Work out the finished part from the listing and answer in its coordinate system (mm). Face numbers are marked on the shaded views. A direction names the side the tool comes from. Round coordinates to 2 decimals unless told otherwise and drop trailing zeros. Loops run counter-clockwise (first coordinate to the right, second up) from the corner with the lowest first, then second, coordinate; pieces in that order, holes last. Notation, with made-up numbers: (19.5, 70.25) -> (31.5, 70.25) arc R13 cw to (31.5, 91.25) -> close; hole circle Ø3 at (38, 84). An arc over 180 degrees is marked (long way). Use one line per item in the form item = value.
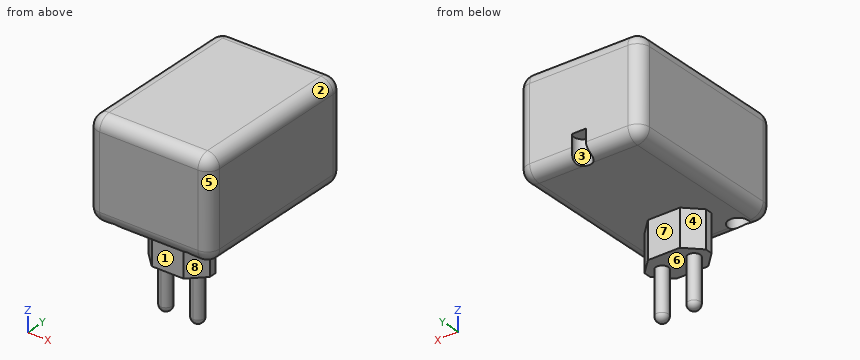
```python
from build123d import *

# Parameters (mm, degrees)
F0_W          = 50
F0_H          = 70
F1_DEPTH      = 40
F3_DEPTH      = 15
F4_SIZE       = 6
F6_DEPTH      = 20
F7_DEPTH      = 20
F8_R          = 2.5
F10_DEPTH     = 10
F12_DEPTH     = 8
F13_T1_DEPTH  = 60
F13_T3_DEPTH  = 30
F13_T5_DEPTH  = 29.6276373277
F13_T7_DEPTH  = 29.6276373277
F13_T9_DEPTH  = 40
F13_S13_W     = 5
F13_S13_H     = 5
F13_T14_DEPTH = 5
F13_S19_W     = 5
F13_S19_H     = 5
F13_T20_DEPTH = 5
F13_S25_W     = 5
F13_S25_H     = 5
F13_T26_DEPTH = 5
F13_S31_W     = 5
F13_S31_H     = 5
F13_T32_DEPTH = 5
F13_S37_W     = 5
F13_S37_H     = 5
F13_T38_DEPTH = 5
F13_S43_W     = 5
F13_S43_H     = 5
F13_T44_DEPTH = 5
F13_S49_W     = 5
F13_S49_H     = 5
F13_T50_DEPTH = 5
F13_S55_W     = 5
F13_S55_H     = 5
F13_T56_DEPTH = 5


# Not quite as in the source:
# - a fillet or chamfer that OpenCascade refuses, or shapes differently, is made with other operations: its cross-section is extruded or revolved along the edge and cut away or added


with BuildPart() as f1:
    # F0 (on Top) → F1 (new body)
    with BuildSketch(Plane.XY):
        Rectangle(F0_W, F0_H)
    extrude(amount=F1_DEPTH)

    # F2 (on face) → F3 (join)
    with BuildSketch(Plane(origin=(0, 0, 0), x_dir=(1, 0, 0), z_dir=(0, 0, -1))):
        Polygon((-12.5, 25), (-12.5, 20), (-12.5, 10), (12.5, 10), (12.5, 17.5), (12.5, 25), align=None)
    extrude(amount=F3_DEPTH)

    # F4
    f4_edges = [f1.edges().sort_by_distance(p)[0] for p in [
        (-12.5, -25, -7.5),
        (-12.5, -10, -7.5),
        (12.5, -10, -7.5),
        (12.5, -25, -7.5),
    ]]
    chamfer(f4_edges, length=F4_SIZE)

    # F5 (on face) → F6 (join)
    with BuildSketch(Plane(origin=(0, 0, -15), x_dir=(1, 0, 0), z_dir=(0, 0, -1))):
        with BuildLine():
            ThreePointArc((-4, 17.5), (-4.732233047, 19.267766953), (-6.5, 20))
            ThreePointArc((-6.5, 20), (-8.267766953, 15.732233047), (-4, 17.5))
        make_face()
    extrude(amount=F6_DEPTH)

    # F5 (on face) → F7 (join)
    with BuildSketch(Plane(origin=(0, 0, -15), x_dir=(1, 0, 0), z_dir=(0, 0, -1))):
        with BuildLine():
            ThreePointArc((9, 17.5), (8.267766953, 19.267766953), (6.5, 20))
            ThreePointArc((6.5, 20), (4.732233047, 15.732233047), (9, 17.5))
        make_face()
    extrude(amount=F7_DEPTH)

    # F8
    f8_edges = [f1.edges().sort_by_distance(p)[0] for p in [
        (-9, -17.5, -35),
        (4, -17.5, -35),
    ]]
    fillet(f8_edges, radius=F8_R)

    # F9 (on face) → F10 (cut)
    with BuildSketch(Plane(origin=(0, 0, 0), x_dir=(1, 0, 0), z_dir=(0, 0, -1))):
        with BuildLine():
            Line((-2.8723626723, -35), (2.8723626723, -35))
            ThreePointArc((2.8723626723, -35), (0, -29.4152137969), (-2.8723626723, -35))
        make_face()
    extrude(amount=-F10_DEPTH, mode=Mode.SUBTRACT)

    # F11 (on face) → F12 (cut)
    with BuildSketch(Plane(origin=(0, 0, 0), x_dir=(1, 0, 0), z_dir=(0, 0, -1))):
        with BuildLine():
            ThreePointArc((11, 29.8445560038), (15, 25.8445560038), (19, 29.8445560038))
            Line((19, 29.8445560038), (15, 29.8445560038))
            Line((15, 29.8445560038), (11, 29.8445560038))
        make_face()
        with BuildLine():
            Line((-15, 29.8445560038), (-11, 29.8445560038))
            ThreePointArc((-11, 29.8445560038), (-15, 33.8445560038), (-19, 29.8445560038))
            Line((-19, 29.8445560038), (-15, 29.8445560038))
        make_face()
        with BuildLine():
            ThreePointArc((-19, 29.8445560038), (-15, 25.8445560038), (-11, 29.8445560038))
            Line((-11, 29.8445560038), (-15, 29.8445560038))
            Line((-15, 29.8445560038), (-19, 29.8445560038))
        make_face()
        with BuildLine():
            Line((15, 29.8445560038), (19, 29.8445560038))
            ThreePointArc((19, 29.8445560038), (15, 33.8445560038), (11, 29.8445560038))
            Line((11, 29.8445560038), (15, 29.8445560038))
        make_face()
    extrude(amount=-F12_DEPTH, mode=Mode.SUBTRACT)

    # F13: fillet of radius 5 on 13 edges, made by hand

    # F13_s2 → F13_t1 (cut)
    with BuildSketch(Plane.XZ.offset(-30)):
        with BuildLine():
            ThreePointArc((20, 0), (23.5355339059, 1.4644660941), (25, 5))
            Line((25, 5), (25, 0))
            Line((25, 0), (20, 0))
        make_face()
        with BuildLine():
            ThreePointArc((25, 35), (23.5355339059, 38.5355339059), (20, 40))
            Line((20, 40), (25, 40))
            Line((25, 40), (25, 35))
        make_face()
        with BuildLine():
            ThreePointArc((-20, 0), (-23.5355339059, 1.4644660941), (-25, 5))
            Line((-25, 5), (-25, 0))
            Line((-25, 0), (-20, 0))
        make_face()
        with BuildLine():
            ThreePointArc((-25, 35), (-23.5355339059, 38.5355339059), (-20, 40))
            Line((-20, 40), (-25, 40))
            Line((-25, 40), (-25, 35))
        make_face()
    extrude(amount=F13_T1_DEPTH, mode=Mode.SUBTRACT)

    # F13_s4 → F13_t3 (cut)
    with BuildSketch(Plane.XY.offset(5)):
        with BuildLine():
            ThreePointArc((20, -35), (23.5355339059, -33.5355339059), (25, -30))
            Line((25, -30), (25, -35))
            Line((25, -35), (20, -35))
        make_face()
        with BuildLine():
            ThreePointArc((20, 35), (23.5355339059, 33.5355339059), (25, 30))
            Line((25, 30), (25, 35))
            Line((25, 35), (20, 35))
        make_face()
        with BuildLine():
            ThreePointArc((-25, -30), (-23.5355339059, -33.5355339059), (-20, -35))
            Line((-20, -35), (-25, -35))
            Line((-25, -35), (-25, -30))
        make_face()
        with BuildLine():
            ThreePointArc((-25, 30), (-23.5355339059, 33.5355339059), (-20, 35))
            Line((-20, 35), (-25, 35))
            Line((-25, 35), (-25, 30))
        make_face()
    extrude(amount=F13_T3_DEPTH, mode=Mode.SUBTRACT)

    # F13_s6 → F13_t5 (cut)
    with BuildSketch(Plane.YZ.offset(-9.6276373277)):
        with BuildLine():
            ThreePointArc((30, 0), (33.5355339059, 1.4644660941), (35, 5))
            Line((35, 5), (35, 0))
            Line((35, 0), (30, 0))
        make_face()
    extrude(amount=F13_T5_DEPTH, mode=Mode.SUBTRACT)

    # F13_s8 → F13_t7 (cut)
    with BuildSketch(Plane.YZ.offset(-20)):
        with BuildLine():
            ThreePointArc((30, 0), (33.5355339059, 1.4644660941), (35, 5))
            Line((35, 5), (35, 0))
            Line((35, 0), (30, 0))
        make_face()
    extrude(amount=F13_T7_DEPTH, mode=Mode.SUBTRACT)

    # F13_s10 → F13_t9 (cut)
    with BuildSketch(Plane.YZ.offset(-20)):
        with BuildLine():
            ThreePointArc((-30, 0), (-33.5355339059, 1.4644660941), (-35, 5))
            Line((-35, 5), (-35, 0))
            Line((-35, 0), (-30, 0))
        make_face()
        with BuildLine():
            ThreePointArc((-35, 35), (-33.5355339059, 38.5355339059), (-30, 40))
            Line((-30, 40), (-35, 40))
            Line((-35, 40), (-35, 35))
        make_face()
        with BuildLine():
            ThreePointArc((35, 35), (33.5355339059, 38.5355339059), (30, 40))
            Line((30, 40), (35, 40))
            Line((35, 40), (35, 35))
        make_face()
    extrude(amount=F13_T9_DEPTH, mode=Mode.SUBTRACT)


with BuildPart() as f13_tool12:
    # F13_s13 → F13_t14 (new body)
    with BuildSketch(Plane.XZ.offset(30)):
        with Locations((22.5, 2.5)):
            Rectangle(F13_S13_W, F13_S13_H)
    extrude(amount=F13_T14_DEPTH)

    # F13_s15 → F13_t16 (revolve, cut)
    with BuildSketch(Plane(origin=(20, -30, 5), x_dir=(-0.7071067812, 0, 0.7071067812), z_dir=(0.7071067812, 0, 0.7071067812))):
        with BuildLine():
            ThreePointArc((0, -5), (5, 0), (0, 5))
            Line((0, 5), (0, -5))
        make_face()
    revolve(axis=Axis((20, -30, 5), (0, -1, 0)), mode=Mode.SUBTRACT)


with BuildPart() as f1_1:
    add(f1.part)

    # F13_t11: cut F13_tool12
    add(f13_tool12.part, mode=Mode.SUBTRACT)


with BuildPart() as f13_tool18:
    # F13_s19 → F13_t20 (new body)
    with BuildSketch(Plane.YZ.offset(20)):
        with Locations((32.5, 2.5)):
            Rectangle(F13_S19_W, F13_S19_H)
    extrude(amount=F13_T20_DEPTH)

    # F13_s21 → F13_t22 (revolve, cut)
    with BuildSketch(Plane(origin=(20, 30, 5), x_dir=(0, -0.7071067812, 0.7071067812), z_dir=(0, 0.7071067812, 0.7071067812))):
        with BuildLine():
            ThreePointArc((0, -5), (5, 0), (0, 5))
            Line((0, 5), (0, -5))
        make_face()
    revolve(axis=Axis((20, 30, 5), (1, 0, 0)), mode=Mode.SUBTRACT)


with BuildPart() as f1_2:
    add(f1_1.part)

    # F13_t17: cut F13_tool18
    add(f13_tool18.part, mode=Mode.SUBTRACT)


with BuildPart() as f13_tool24:
    # F13_s25 → F13_t26 (new body)
    with BuildSketch(Plane.XZ.offset(30)):
        with Locations((22.5, 37.5)):
            Rectangle(F13_S25_W, F13_S25_H)
    extrude(amount=F13_T26_DEPTH)

    # F13_s27 → F13_t28 (revolve, cut)
    with BuildSketch(Plane(origin=(20, -30, 35), x_dir=(-0.7071067812, 0, -0.7071067812), z_dir=(-0.7071067812, 0, 0.7071067812))):
        with BuildLine():
            ThreePointArc((0, -5), (5, 0), (0, 5))
            Line((0, 5), (0, -5))
        make_face()
    revolve(axis=Axis((20, -30, 35), (0, -1, 0)), mode=Mode.SUBTRACT)


with BuildPart() as f1_3:
    add(f1_2.part)

    # F13_t23: cut F13_tool24
    add(f13_tool24.part, mode=Mode.SUBTRACT)


with BuildPart() as f13_tool30:
    # F13_s31 → F13_t32 (new body)
    with BuildSketch(Plane.YZ.offset(20)):
        with Locations((32.5, 37.5)):
            Rectangle(F13_S31_W, F13_S31_H)
    extrude(amount=F13_T32_DEPTH)

    # F13_s33 → F13_t34 (revolve, cut)
    with BuildSketch(Plane(origin=(20, 30, 35), x_dir=(0, -0.7071067812, -0.7071067812), z_dir=(0, -0.7071067812, 0.7071067812))):
        with BuildLine():
            ThreePointArc((0, -5), (5, 0), (0, 5))
            Line((0, 5), (0, -5))
        make_face()
    revolve(axis=Axis((20, 30, 35), (1, 0, 0)), mode=Mode.SUBTRACT)


with BuildPart() as f1_4:
    add(f1_3.part)

    # F13_t29: cut F13_tool30
    add(f13_tool30.part, mode=Mode.SUBTRACT)


with BuildPart() as f13_tool36:
    # F13_s37 → F13_t38 (new body)
    with BuildSketch(Plane.XY.offset(5)):
        with Locations((-22.5, 32.5)):
            Rectangle(F13_S37_W, F13_S37_H)
    extrude(amount=-F13_T38_DEPTH)

    # F13_s39 → F13_t40 (revolve, cut)
    with BuildSketch(Plane(origin=(-20, 30, 5), x_dir=(0.7071067812, -0.7071067812, 0), z_dir=(0.7071067812, 0.7071067812, 0))):
        with BuildLine():
            ThreePointArc((0, -5), (5, 0), (0, 5))
            Line((0, 5), (0, -5))
        make_face()
    revolve(axis=Axis((-20, 30, 5), (0, 0, -1)), mode=Mode.SUBTRACT)


with BuildPart() as f1_5:
    add(f1_4.part)

    # F13_t35: cut F13_tool36
    add(f13_tool36.part, mode=Mode.SUBTRACT)


with BuildPart() as f13_tool42:
    # F13_s43 → F13_t44 (new body)
    with BuildSketch(Plane.XZ.offset(30)):
        with Locations((-22.5, 2.5)):
            Rectangle(F13_S43_W, F13_S43_H)
    extrude(amount=F13_T44_DEPTH)

    # F13_s45 → F13_t46 (revolve, cut)
    with BuildSketch(Plane(origin=(-20, -30, 5), x_dir=(0.7071067812, 0, 0.7071067812), z_dir=(0.7071067812, 0, -0.7071067812))):
        with BuildLine():
            ThreePointArc((0, -5), (5, 0), (0, 5))
            Line((0, 5), (0, -5))
        make_face()
    revolve(axis=Axis((-20, -30, 5), (0, -1, 0)), mode=Mode.SUBTRACT)


with BuildPart() as f1_6:
    add(f1_5.part)

    # F13_t41: cut F13_tool42
    add(f13_tool42.part, mode=Mode.SUBTRACT)


with BuildPart() as f13_tool48:
    # F13_s49 → F13_t50 (new body)
    with BuildSketch(Plane.XZ.offset(30)):
        with Locations((-22.5, 37.5)):
            Rectangle(F13_S49_W, F13_S49_H)
    extrude(amount=F13_T50_DEPTH)

    # F13_s51 → F13_t52 (revolve, cut)
    with BuildSketch(Plane(origin=(-20, -30, 35), x_dir=(0.7071067812, 0, -0.7071067812), z_dir=(-0.7071067812, 0, -0.7071067812))):
        with BuildLine():
            ThreePointArc((0, -5), (5, 0), (0, 5))
            Line((0, 5), (0, -5))
        make_face()
    revolve(axis=Axis((-20, -30, 35), (0, -1, 0)), mode=Mode.SUBTRACT)


with BuildPart() as f1_7:
    add(f1_6.part)

    # F13_t47: cut F13_tool48
    add(f13_tool48.part, mode=Mode.SUBTRACT)


with BuildPart() as f13_tool54:
    # F13_s55 → F13_t56 (new body)
    with BuildSketch(Plane.XY.offset(35)):
        with Locations((-22.5, 32.5)):
            Rectangle(F13_S55_W, F13_S55_H)
    extrude(amount=F13_T56_DEPTH)

    # F13_s57 → F13_t58 (revolve, cut)
    with BuildSketch(Plane(origin=(-20, 30, 35), x_dir=(0.7071067812, -0.7071067812, 0), z_dir=(-0.7071067812, -0.7071067812, 0))):
        with BuildLine():
            ThreePointArc((0, -5), (5, 0), (0, 5))
            Line((0, 5), (0, -5))
        make_face()
    revolve(axis=Axis((-20, 30, 35), (0, 0, 1)), mode=Mode.SUBTRACT)


with BuildPart() as f1_8:
    add(f1_7.part)

    # F13_t53: cut F13_tool54
    add(f13_tool54.part, mode=Mode.SUBTRACT)


solid = f1_8.part
```
(1) For a pull along Y with two mould halves and no side action, classify the marked faces 1, 2 and 3 as +Y half, -Y half, draft (parallel to the pull), parting line (faces both ways), or undercut.
Completed:
face_1 = -Y half
face_2 = draft
face_3 = undercut
(2) Find section D-D, the plane x = -8. Write down the section's boundary in (y, z).
Completed:
outline = (-35, 5) arc R5 ccw to (-30, 0) -> (-23.5, 0) -> (-23.5, -15) -> (-19.5, -15) -> (-19.5, -32.5) arc R2 ccw to (-15.5, -32.5) -> (-15.5, -15) -> (-11.5, -15) -> (-11.5, 0) -> (30, 0) arc R5 ccw to (35, 5) -> (35, 35) arc R5 ccw to (30, 40) -> (-30, 40) arc R5 ccw to (-35, 35) -> close
(3) For the marked faces 4, 5, 6, 7 and 8, determine the directions among +Z, -Z, +X, -X, +Y, -Y from which every point of the face is accessible in a straight line to the end or side of a thin tool.
Completed:
face_4 = -Z, -X, +Y
face_5 = +Z, -Z, +X, -Y
face_6 = -Z
face_7 = -Z, +X, -X, +Y
face_8 = -Z, +X, -Y
(4) Find section B-B, the plane y = 23.5. Write down the section's boundary in (x, z).
Completed:
outline = (-25, 5) arc R5 ccw to (-20, 0) -> (20, 0) arc R5 ccw to (25, 5) -> (25, 35) arc R5 ccw to (20, 40) -> (-20, 40) arc R5 ccw to (-25, 35) -> close
(5) Consider L1, parallel to X at y = -27, z = 5; L2, parallel to Y at x = 0, z = 6.25; L3, parallel to Z at x = -0.5, y = -15. Determine where each line is inside the solid, lowest interval first.
Completed:
L1 = -25 to -17.81, -12.19 to 12.19, 17.81 to 25
L2 = -35 to 29.42
L3 = -15 to 40
(6) Find section C-C, the plane z = -9. Write down the section's boundary in (x, y).
Completed:
outline = (-12.5, -19) -> (-6.5, -25) -> (6.5, -25) -> (12.5, -19) -> (12.5, -16) -> (6.5, -10) -> (-6.5, -10) -> (-12.5, -16) -> close
(7) Given P1, Ø10.5, axis at x = 3, z = -5.5, coming from the +Y side; P2, Ø2.5, axis at x = 13.5, y = -31, coming from the -Z side; P3, Ø4, axis at x = -10.5, z = -10.5, coming from the +Y side, each flat-ended and moving along its own axis, determine where each tip first touches the part or whether it passes through.
Completed:
P1 = -10
P2 = 8
P3 = -12
(8) Find section A-A, the plane x = 10. Write down the section's boundary in (y, z).
Completed:
outline = (-35, 5) arc R5 ccw to (-30, 0) -> (-21.5, 0) -> (-21.5, -15) -> (-13.5, -15) -> (-13.5, 0) -> (30, 0) arc R5 ccw to (35, 5) -> (35, 35) arc R5 ccw to (30, 40) -> (-30, 40) arc R5 ccw to (-35, 35) -> close
